Read the model definition and answer for the solid it produces. Units are mm, in the model's axes. A direction names the side the tool comes from. Give positions to 0.01 mm unless a question says otherwise; leave off trailing zeros. Loops run counter-clockwise (first coordinate to the right, second up) from the corner with the lowest first, then second, coordinate; pieces in that order, holes last. Notation, with made-up numbers: (48, -11.5) -> (96, -11.5) arc R27 cw to (96, 23.5) -> close; hole circle Ø7 at (62.25, 8). An arc over 180 degrees is marked (long way). Write each question's results on one line, items separated by ' | '. Start each with the question number.
Item 1: Section D-D on y = 21 is taken. Write down the section's boundary in (x, z).
Item 2: Which of the six approach directions +Z, -Z, +X, -X, +Y, -Y give full straight-line access (tool end or side, diameter ignored) to faces 4 (the flat face through (70, 15, 20)), 5 (the flat face through (61, 25, 35))?
Item 3: Determine the mould class of faces 1 (the cylindrical face through (4.6, 15.57, 34.93)), 2 (the cylindrical face through (66.99, 37.15, 20.28)), 3 (the flat face through (35, 0, 20)) for opening direction X: +X half, -X half, draft (parallel to the pull), parting line (faces both ways), or undercut.
Item 4: Section C-C on z = 25 is taken. Write down the section's boundary in (x, y).
Item 5: This flat-tipped pin is pushed along its axis until it touches: P1, Ø8, axis at x = 21.5, y = 22, coming from the +Z side. Where does it stop, or does it pass through?
Item 6: Find the intervals of material crossed by line 1 (Y direction, x = 32, z = 37); line 2 (Z direction, x = 52.5, y = 24); line 3 (Y direction, x = 9.5, z = 13), in increasing order.
Item 7: Section B-B on x = 35 is taken. Write down the section's boundary in (y, z), and give its area (3 significant figures).
Item 8: Section A-A on y = 7 is taken. Write down the section's boundary in (x, z).
```python
from build123d import *

# Parameters (mm, degrees)
SKETCH1_W           = 70
SKETCH1_H           = 40
BOSS_EXTRUDE1_DEPTH = 40
CUT_EXTRUDE1_DEPTH  = 10
CUT_EXTRUDE2_DEPTH  = 10
CUT_EXTRUDE3_DEPTH  = 10
SKETCH5_W           = 10
SKETCH5_H           = 10
CUT_EXTRUDE4_DEPTH  = 10
SKETCH6_W           = 10
SKETCH6_H           = 10
CUT_EXTRUDE5_DEPTH  = 10
FILLET21_R          = 2
FILLET22_R          = 10
SKETCH7_R           = 1
CUT_EXTRUDE6_DEPTH  = 10


with BuildPart() as part:
    # Sketch1 → Boss-Extrude1 (new body)
    with BuildSketch(Plane.XY):
        with Locations((35, 20)):
            Rectangle(SKETCH1_W, SKETCH1_H)
    extrude(amount=BOSS_EXTRUDE1_DEPTH)

    # Sketch2 → Cut-Extrude1 (cut)
    with BuildSketch(Plane.XY.offset(40)):
        Polygon((30, 20), (30, 30), (40, 30), (40, 20), (40, 10), (30, 10), align=None)
    extrude(amount=-CUT_EXTRUDE1_DEPTH, mode=Mode.SUBTRACT)

    # Sketch3 → Cut-Extrude2 (cut)
    with BuildSketch(Plane.XY.offset(40)):
        Polygon((27, 12.5), (17, 12.5), (17, 27.5), (27, 27.5), (27, 15), align=None)
    extrude(amount=-CUT_EXTRUDE2_DEPTH, mode=Mode.SUBTRACT)

    # Sketch4 → Cut-Extrude3 (cut)
    with BuildSketch(Plane.XY.offset(40)):
        Polygon((43, 25), (43, 27.5), (53, 27.5), (53, 12.5), (43, 12.5), align=None)
    extrude(amount=-CUT_EXTRUDE3_DEPTH, mode=Mode.SUBTRACT)

    # Sketch5 → Cut-Extrude4 (cut)
    with BuildSketch(Plane.XY.offset(40)):
        with Locations((9, 20)):
            Rectangle(SKETCH5_W, SKETCH5_H)
    extrude(amount=-CUT_EXTRUDE4_DEPTH, mode=Mode.SUBTRACT)

    # Sketch6 → Cut-Extrude5 (cut)
    with BuildSketch(Plane.XY.offset(40)):
        with Locations((61, 20)):
            Rectangle(SKETCH6_W, SKETCH6_H)
    extrude(amount=-CUT_EXTRUDE5_DEPTH, mode=Mode.SUBTRACT)

    # Fillet21
    fillet21_edges = [part.edges().sort_by_distance(p)[0] for p in [
        (30, 30, 35),
        (40, 30, 35),
        (40, 10, 35),
        (30, 10, 35),
        (17, 27.5, 35),
        (27, 27.5, 35),
        (27, 12.5, 35),
        (17, 12.5, 35),
        (53, 27.5, 35),
        (53, 12.5, 35),
        (43, 12.5, 35),
        (43, 27.5, 35),
        (14, 25, 35),
        (14, 15, 35),
        (4, 15, 35),
        (4, 25, 35),
        (66, 25, 35),
        (66, 15, 35),
        (56, 15, 35),
        (56, 25, 35),
    ]]
    fillet(fillet21_edges, radius=FILLET21_R)

    # Fillet22
    fillet22_edges = [part.edges().sort_by_distance(p)[0] for p in [
        (0, 40, 20),
        (70, 40, 20),
    ]]
    fillet(fillet22_edges, radius=FILLET22_R)

    # Sketch7 → Cut-Extrude6 (cut)
    with BuildSketch(Plane.XY.offset(40)):
        with Locations((32, 7)):
            Circle(SKETCH7_R)
        with Locations((35, 7)):
            Circle(SKETCH7_R)
        with Locations((38, 7)):
            Circle(SKETCH7_R)
    extrude(amount=-CUT_EXTRUDE6_DEPTH, mode=Mode.SUBTRACT)


solid = part.part
```
Findings:
1) outline: (0, 0) -> (70, 0) -> (70, 40) -> (66, 40) -> (66, 30) -> (56, 30) -> (56, 40) -> (53, 40) -> (53, 30) -> (43, 30) -> (43, 40) -> (40, 40) -> (40, 30) -> (30, 30) -> (30, 40) -> (27, 40) -> (27, 30) -> (17, 30) -> (17, 40) -> (14, 40) -> (14, 30) -> (4, 30) -> (4, 40) -> (0, 40) -> close
2) face 4: +Z, -Z, +X, +Y, -Y | face 5: +Z
3) face 1: undercut | face 2: +X half | face 3: draft
4) outline: (0, 0) -> (70, 0) -> (70, 30) arc R10 ccw to (60, 40) -> (10, 40) arc R10 ccw to (0, 30) -> close
5) P1: z = 30
6) line 1: 0 to 6, 8 to 10, 30 to 40 | line 2: 0 to 30 | line 3: 0 to 39.99
7) outline: (0, 0) -> (40, 0) -> (40, 40) -> (30, 40) -> (30, 30) -> (10, 30) -> (10, 40) -> (8, 40) -> (8, 30) -> (6, 30) -> (6, 40) -> (0, 40) -> close | area: 1,380 mm2
8) outline: (0, 0) -> (70, 0) -> (70, 40) -> (39, 40) -> (39, 30) -> (37, 30) -> (37, 40) -> (36, 40) -> (36, 30) -> (34, 30) -> (34, 40) -> (33, 40) -> (33, 30) -> (31, 30) -> (31, 40) -> (0, 40) -> close
